Input: part model. Units: mm. Frame: model coordinates. Face numbers are marked on the shaded views. A direction names the side the tool comes from. Coordinates: 2 decimals unless noted, no trailing zeros. Write each loop counter-clockwise with the first axis right and the second up, starting at its lowest first coordinate (ties: lowest second). Pieces come first, ordered by that corner, then holes. Notation, with made-up numbers: (52.25, 39) -> (80.25, 39) arc R18 cw to (80.25, 47) -> close; hole circle Ø1 at (-31, 55). An arc over 180 degrees is marked (long way). Use one line per item in the form item = value. Start each with the question number.
(1) Cut plane B-B on y = 0. Return the cut outline in (x, z), plus the area to 3 significant figures.
(2) Ray query, line 1 along Y through (x, z) = (-13, -2.6); line 2 along Z through (x, y) = (-10, -0.5); line 3 along X through (y, z) = (-3.5, -2.9). Return the intervals inside material, ascending.
(3) Cut plane C-C on z = -0.75. State how many separate pieces and enclosed holes the cut face has, plus the area to 3 significant figures.
(4) First-contact query: pin 1 (0.5 mm diameter, centred on y = -7, z = -1, fed in from -X); pin 2 (0.9 mm diameter, centred on y = 2, z = -1, fed in from -X); pin 3 (2 mm diameter, centred on x = -14, y = -1, fed in from +Z); pin 4 (4 mm diameter, centred on x = 8.11, y = 0, fed in from +Z). Flat tips, straight axial feed; report the tip coordinate or a pass-through.
(5) Cut plane D-D on x = -2. Return the cut outline in (y, z), plus the area to 3 significant figures.
(6) Cut plane A-A on z = -2.65. Return the cut outline in (x, y).
(7) Pull-direction query (X, two-part tool) for the marked faces 3, 4 and 5; classes: released by +X, released by -X, zero draft, split by the parting line, or undercut.
(8) Set-up query: the marked faces 1 and 2. Return all of +Z, -Z, +X, -X, +Y, -Y with unobstructed straight access to the full face (end or side cutting, diameter ignored); none if empty.
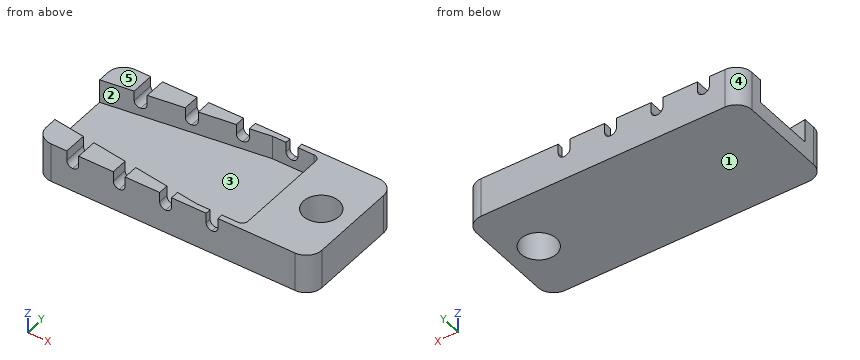
```python
from build123d import *

# Parameters (mm, degrees)
F0_W     = 1.5
F0_H     = 0.7
F0_R     = 2.25
F0_H_2   = 13.6
F0_W_2   = 2.8
F1_DEPTH = 5
F2_DEPTH = 3
F3_DEPTH = 2
F4_R     = 0.74999
F5_R     = 2


# Not quite as in the source:
# - a fillet or chamfer is up to 0.001 mm smaller than in the source, because OpenCascade refuses the exact size


with BuildPart() as f1:
    # F0 (on Top) → F1 (new body)
    with BuildSketch(Plane.XY):
        Polygon((-18.8879279066, 7.5), (-22.8879279066, 7.5), (-22.8879279066, 4), (-18.8879279066, 4.56), align=None)
        Polygon((-17.3879279066, 7.5), (-18.8879279066, 7.5), (-18.8879279066, 4.56), (-17.3879279066, 4.77), align=None)
        Polygon((-18.8879279066, 4.56), (-22.8879279066, 4), (-22.8879279066, -4), (-18.8879279066, -4.56), align=None)
        Polygon((-12.9879279066, 7.5), (-17.3879279066, 7.5), (-17.3879279066, 4.77), (-12.9879279066, 5.386), align=None)
        Polygon((-18.8879279066, -4.56), (-22.8879279066, -4), (-22.8879279066, -7.5), (-18.8879279066, -7.5), align=None)
        Polygon((-11.4879279066, 7.5), (-12.9879279066, 7.5), (-12.9879279066, 5.386), (-11.4879279066, 5.596), align=None)
        Polygon((-17.3879279066, -4.77), (-18.8879279066, -4.56), (-18.8879279066, -7.5), (-17.3879279066, -7.5), align=None)
        Polygon((-7.0879279066, 7.5), (-11.4879279066, 7.5), (-11.4879279066, 5.596), (-7.0879279066, 6.212), align=None)
        Polygon((-12.9879279066, -5.386), (-17.3879279066, -4.77), (-17.3879279066, -7.5), (-12.9879279066, -7.5), align=None)
        Polygon((-5.5879279066, 7.5), (-7.0879279066, 7.5), (-7.0879279066, 6.212), (-5.5879279066, 6.422), align=None)
        Polygon((-11.4879279066, -5.596), (-12.9879279066, -5.386), (-12.9879279066, -7.5), (-11.4879279066, -7.5), align=None)
        Polygon((-1.1879279066, 7.5), (-5.5879279066, 7.5), (-5.5879279066, 6.422), (-2.8879279066, 6.8), (-1.1879279066, 6.8), align=None)
        Polygon((-7.0879279066, -6.212), (-11.4879279066, -5.596), (-11.4879279066, -7.5), (-7.0879279066, -7.5), align=None)
        with Locations((-0.4379279066, 7.15)):
            Rectangle(F0_W, F0_H)
        Polygon((-5.5879279066, -6.422), (-7.0879279066, -6.212), (-7.0879279066, -7.5), (-5.5879279066, -7.5), align=None)
        Polygon((12.1120720934, 7.5), (0.3120720934, 7.5), (0.3120720934, 6.8), (3.1120720934, 6.8), (3.1120720934, -6.8), (0.3120720934, -6.8), (0.3120720934, -7.5), (12.1120720934, -7.5), align=None)
        with Locations((8.1120720934, 0)):
            Circle(F0_R, mode=Mode.SUBTRACT)
        Polygon((-2.8879279066, -6.8), (-5.5879279066, -6.422), (-5.5879279066, -7.5), (-1.1879279066, -7.5), (-1.1879279066, -6.8), align=None)
        with Locations((-0.4379279066, -7.15)):
            Rectangle(F0_W, F0_H)
        with Locations((-0.4379279066, 0)):
            Rectangle(F0_W, F0_H_2)
        Polygon((-5.5879279066, 6.422), (-7.0879279066, 6.212), (-7.0879279066, -6.212), (-5.5879279066, -6.422), align=None)
        Polygon((-17.3879279066, 4.77), (-18.8879279066, 4.56), (-18.8879279066, -4.56), (-17.3879279066, -4.77), align=None)
        Polygon((-12.9879279066, 5.386), (-17.3879279066, 4.77), (-17.3879279066, -4.77), (-12.9879279066, -5.386), align=None)
        Polygon((-7.0879279066, 6.212), (-11.4879279066, 5.596), (-11.4879279066, -5.596), (-7.0879279066, -6.212), align=None)
        Polygon((-11.4879279066, 5.596), (-12.9879279066, 5.386), (-12.9879279066, -5.386), (-11.4879279066, -5.596), align=None)
        Polygon((-2.8879279066, 6.8), (-5.5879279066, 6.422), (-5.5879279066, -6.422), (-2.8879279066, -6.8), (-1.1879279066, -6.8), (-1.1879279066, 6.8), align=None)
        with Locations((1.7120720934, 0)):
            Rectangle(F0_W_2, F0_H_2)
    extrude(amount=-F1_DEPTH)

    # F0 (on Top) → F2 (cut)
    with BuildSketch(Plane.XY):
        Polygon((-18.8879279066, 4.56), (-22.8879279066, 4), (-22.8879279066, -4), (-18.8879279066, -4.56), align=None)
        Polygon((-17.3879279066, 4.77), (-18.8879279066, 4.56), (-18.8879279066, -4.56), (-17.3879279066, -4.77), align=None)
        Polygon((-12.9879279066, 5.386), (-17.3879279066, 4.77), (-17.3879279066, -4.77), (-12.9879279066, -5.386), align=None)
        Polygon((-11.4879279066, 5.596), (-12.9879279066, 5.386), (-12.9879279066, -5.386), (-11.4879279066, -5.596), align=None)
        Polygon((-7.0879279066, 6.212), (-11.4879279066, 5.596), (-11.4879279066, -5.596), (-7.0879279066, -6.212), align=None)
        Polygon((-5.5879279066, 6.422), (-7.0879279066, 6.212), (-7.0879279066, -6.212), (-5.5879279066, -6.422), align=None)
        Polygon((-2.8879279066, 6.8), (-5.5879279066, 6.422), (-5.5879279066, -6.422), (-2.8879279066, -6.8), (-1.1879279066, -6.8), (-1.1879279066, 6.8), align=None)
        with Locations((-0.4379279066, 0)):
            Rectangle(F0_W, F0_H_2)
        with Locations((1.7120720934, 0)):
            Rectangle(F0_W_2, F0_H_2)
    extrude(amount=-F2_DEPTH, mode=Mode.SUBTRACT)

    # F0 (on Top) → F3 (cut)
    with BuildSketch(Plane.XY):
        Polygon((-17.3879279066, 7.5), (-18.8879279066, 7.5), (-18.8879279066, 4.56), (-17.3879279066, 4.77), align=None)
        Polygon((-11.4879279066, 7.5), (-12.9879279066, 7.5), (-12.9879279066, 5.386), (-11.4879279066, 5.596), align=None)
        Polygon((-5.5879279066, 7.5), (-7.0879279066, 7.5), (-7.0879279066, 6.212), (-5.5879279066, 6.422), align=None)
        with Locations((-0.4379279066, -7.15)):
            Rectangle(F0_W, F0_H)
        Polygon((-17.3879279066, -4.77), (-18.8879279066, -4.56), (-18.8879279066, -7.5), (-17.3879279066, -7.5), align=None)
        Polygon((-11.4879279066, -5.596), (-12.9879279066, -5.386), (-12.9879279066, -7.5), (-11.4879279066, -7.5), align=None)
        Polygon((-5.5879279066, -6.422), (-7.0879279066, -6.212), (-7.0879279066, -7.5), (-5.5879279066, -7.5), align=None)
        with Locations((-0.4379279066, 7.15)):
            Rectangle(F0_W, F0_H)
    extrude(amount=-F3_DEPTH, mode=Mode.SUBTRACT)

    # F4 (radius 0.75 in the source; OpenCascade refuses exactly that, so slightly less here)
    f4_edges = [f1.edges().sort_by_distance(p)[0] for p in [
        (-17.387928, -6.135, -2),
        (-11.487928, -6.548, -2),
        (-5.587928, -6.961, -2),
        (0.312072, -7.15, -2),
        (-18.887928, -6.03, -2),
        (-12.987928, -6.443, -2),
        (-7.087928, -6.856, -2),
        (-1.187928, -7.15, -2),
        (-18.887928, 6.03, -2),
        (-12.987928, 6.443, -2),
        (-7.087928, 6.856, -2),
        (-1.187928, 7.15, -2),
        (-17.387928, 6.135, -2),
        (-11.487928, 6.548, -2),
        (-5.587928, 6.961, -2),
        (0.312072, 7.15, -2),
        (3.112072, 6.8, -1.5),
        (3.112072, -6.8, -1.5),
    ]]
    fillet(f4_edges, radius=F4_R)

    # F5
    f5_edges = [f1.edges().sort_by_distance(p)[0] for p in [
        (-22.887928, -7.5, -2.5),
        (-22.887928, 7.5, -2.5),
        (12.112072, -7.5, -2.5),
        (12.112072, 7.5, -2.5),
    ]]
    fillet(f5_edges, radius=F5_R)


solid = f1.part
```
Values:
q1.outline = (-22.89, -5) -> (5.86, -5) -> (5.86, 0) -> (3.11, 0) -> (3.11, -3) -> (-22.89, -3) -> close; (10.36, -5) -> (12.11, -5) -> (12.11, 0) -> (10.36, 0) -> close
q1.area = 74.5 mm2
q2.line_1 = -7.5 to -5.38, 5.38 to 7.5
q2.line_2 = -5 to -3
q2.line_3 = 3.11 to 12.11
q3.separate_pieces = 9
q3.enclosed_holes = 1
q3.area = 188 mm2
q4.pin_1 = -22.45
q4.pin_2 = 3.11
q4.pin_3 = -3
q4.pin_4 = through
q5.outline = (-7.5, -5) -> (7.5, -5) -> (7.5, 0) -> (6.8, 0) -> (6.8, -3) -> (-6.8, -3) -> (-6.8, 0) -> (-7.5, 0) -> close
q5.area = 34.2 mm2
q6.outline = (-22.89, -5.5) arc R2 ccw to (-20.89, -7.5) -> (10.11, -7.5) arc R2 ccw to (12.11, -5.5) -> (12.11, 5.5) arc R2 ccw to (10.11, 7.5) -> (-20.89, 7.5) arc R2 ccw to (-22.89, 5.5) -> (-22.89, 4) -> (-2.89, 6.8) -> (2.36, 6.8) arc R0.75 cw to (3.11, 6.05) -> (3.11, -6.05) arc R0.75 cw to (2.36, -6.8) -> (-2.89, -6.8) -> (-22.89, -4) -> close; hole circle Ø4.5 at (8.11, 0)
q7.face_3 = undercut
q7.face_4 = released by -X
q7.face_5 = zero draft
q8.face_1 = -Z, +X, -X, +Y, -Y
q8.face_2 = +Z
